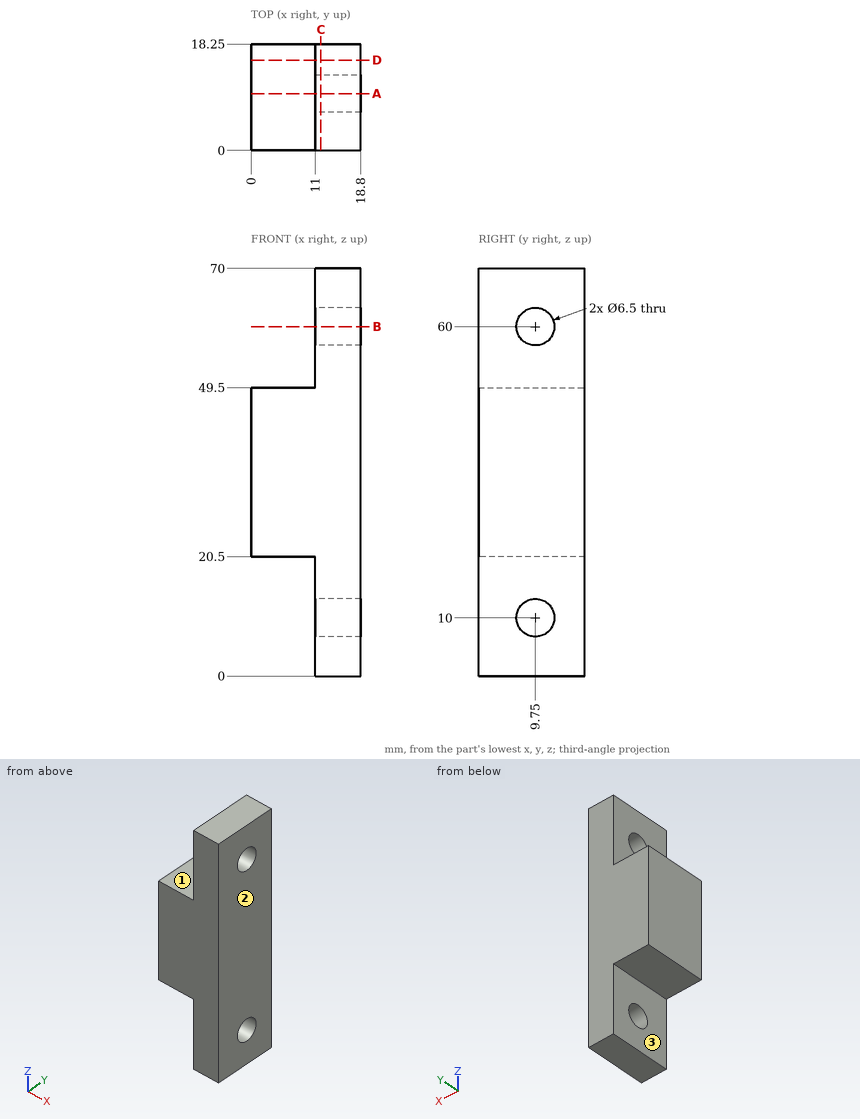
Geometry: see drawing. Coordinates: mm, zero at the bounding-box minimum. A direction names the side the tool comes from. Give positions to 0.01 mm unless a question says otherwise; leave off trailing zeros. Write each loop counter-clockwise with the first axis right and the second up, starting at its lowest first coordinate (ties: lowest second). Pieces come first, ordered by that corner, then holes. Notation, with made-up numbers: (31, -28.75) - (75, -28.75) arc R23 cw to (75, 2.25) - close; hole circle Ø5 at (19.25, 88.5). An arc over 180 degrees is marked (long way). Return JSON: item names as keys, results as strings. Group by question number.
1) Set-up query: the marked faces 1, 2 and 3. Return all of +Z, -Z, +X, -X, +Y, -Y with unobstructed straight access to the full face (end or side cutting, diameter ignored); none if empty.
2) Section D-D on y = 15.5. Return the cut outline in (x, z).
3) Section A-A on y = 9.75. Return the cut outline in (x, z).
4) Section B-B on z = 60. Return the cut outline in (x, y), plus the area to 4 significant figures.
5) Section C-C on x = 12. Return the cut outline in (y, z), plus the area to 3 significant figures.
6) First-contact query: P1, Ø5, axis at y = 9.75, z = 60, coming from the -X side; P2, Ø5.5, axis at y = 11, z = 5.5, coming from the -X side; P3, Ø5.5, axis at x = 6, y = 12, coming from the +Z side. Flat tips, straight axial feed; report the tip coordinate or a pass-through.
7) Line query: line 1 (Z direction, x = 14, y = 9.75); line 2 (Z direction, x = 13, y = 8); line 3 (Y direction, x = 15.25, z = 10). Output: solid intervals per line, ascending.
Filled in:
{
 "1": {"face 1": "+Z, -X, +Y, -Y", "face 2": "+Z, -Z, +X, +Y, -Y", "face 3": "-Z, -X, +Y, -Y"},
 "2": {"outline": "(0, 20.5) - (11, 20.5) - (11, 0) - (18.8, 0) - (18.8, 70) - (11, 70) - (11, 49.5) - (0, 49.5) - close"},
 "3": {"outline": "(0, 20.5) - (11, 20.5) - (11, 13.25) - (18.8, 13.25) - (18.8, 56.75) - (11, 56.75) - (11, 49.5) - (0, 49.5) - close; (11, 0) - (18.8, 0) - (18.8, 6.75) - (11, 6.75) - close; (11, 63.25) - (18.8, 63.25) - (18.8, 70) - (11, 70) - close"},
 "4": {"outline": "(11, 0) - (18.8, 0) - (18.8, 6.5) - (11, 6.5) - close; (11, 13) - (18.8, 13) - (18.8, 18.25) - (11, 18.25) - close", "area": "91.65 mm^2"},
 "5": {"outline": "(0, 0) - (18.25, 0) - (18.25, 70) - (0, 70) - close; hole circle Ø6.5 at (9.75, 10); hole circle Ø6.5 at (9.75, 60)", "area": "1,210 mm^2"},
 "6": {"P1": "passes through", "P2": "stops at x = 11", "P3": "stops at z = 49.5"},
 "7": {"line 1": "z = 0 to 6.75, 13.25 to 56.75, 63.25 to 70", "line 2": "z = 0 to 7.26, 12.74 to 57.26, 62.74 to 70", "line 3": "y = 0 to 6.5, 13 to 18.25"}
}
